Input: dimensioned drawing with shaded views. Units: mm. Origin: part minimum x, y, z. Give positions to 0.01 mm unless a question says otherwise; leave off trailing zeros. Write each loop counter-clockwise with the first axis right and the second up, starting at its lowest first coordinate (ties: lowest second). Pieces come first, ordered by that corner, then holes. Notation, with made-up numbers: (41, -21.75) -> (55, -21.75) arc R16 ccw to (55, -14.75) -> close; hole circle Ø9 at (36.25, 64). An arc over 180 degrees is marked (long way). Return JSON: item names as keys, results as strings. Group by question number.
Item 1: Pin query (flat end, axial travel): P1, Ø1, axis at y = 16, z = 19, coming from the +X side; P2, Ø0.6, axis at x = 11, z = 15, coming from the -Y side; P3, Ø1.6, axis at x = 9, z = 11, coming from the +Y side. Return the tip coordinate at first contact, or that it passes through.
Item 2: Line query: line 1 (Y direction, x = 12.75, z = 3); line 2 (X direction, y = 17.5, z = 10.5). Output: solid intervals per line, ascending. Write a range as [from, to].
Item 3: Section A-A, the plane z = 7.5. Return loops of the section in (x, y).
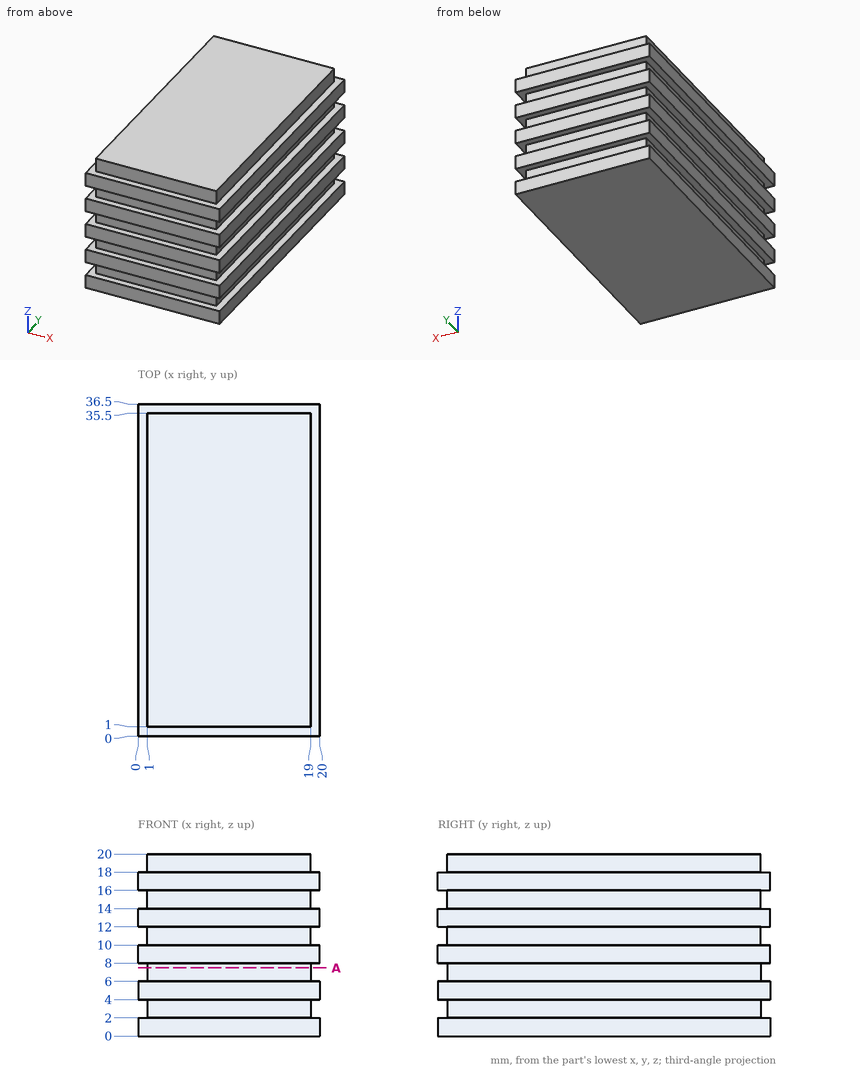
Answer below:
{
 "1": {"P1": "stops at x = 19", "P2": "stops at y = 1", "P3": "stops at y = 35.5"},
 "2": {"line 1": "y = [1, 35.5]", "line 2": "x = [1, 19]"},
 "3": {"outline": "(1, 1) -> (19, 1) -> (19, 35.5) -> (1, 35.5) -> close"}
}
